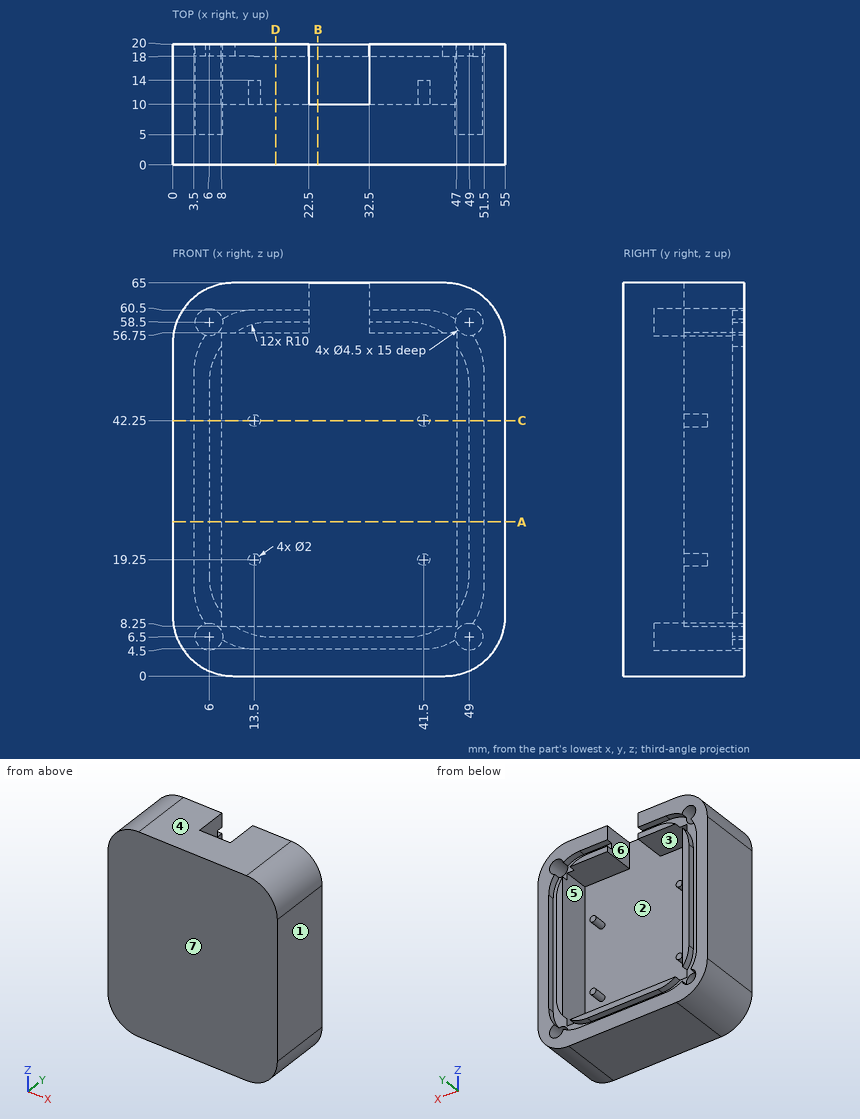
Here's the drawing with two shaded views (mm, measured from the low corner). I have some questions. A direction names the side the tool comes from. Round coordinates to 2 decimals unless told otherwise and drop trailing zeros. Write each loop counter-clockwise with the first axis right and the second up, starting at its lowest first coordinate (ties: lowest second). Pieces come first, ordered by that corner, then holes. Notation, with made-up numbers: M 82.25,41.5 L 93.25,41.5 A28 cw 93.25,78.5 Z; hole C 62.5,-34 d5. An arc over 180 degrees is marked long. Write each question's results on one line, items separated by ' | '. Start each with the question number.
1. On a 3-axis mill with a long thin cutter (end or side, diameter ignored), from which of +Z, -Z, +X, -X, +Y, -Y can I reach the whole of each face in a straight line? I mean the marked faces 5, 6 and 7. Say none if no direction works.
2. Imagine slicing it at A-A on z = 25.5. List the corners of the cut face in (x, y) for me, and give its area (3 significant figures).
3. I need wall thicknesses on L1, parallel to X at y = 14.75, z = 6.5; L2, parallel to Z at x = 49, y = 8.5; L3, parallel to X at y = 19, z = 50. Which ranges of each line are inside material? Lowest first, please. Write a range as from..to.
4. I'm going to push flat-ended pins straight in: pin 1 Ø2 at (x, z) = (6, 5.5) entering from +Y; pin 2 Ø0.6 at (x, z) = (41.5, 19) entering from +Y; pin 3 Ø3.5 at (x, z) = (48, 57.5) entering from +Y. Where does each tip first touch, or does it pass through?
5. Thinking about a two-plate mould opening in Z: for the marked faces 1, 2, 3 and 4, which applies, +Z half, -Z half, draft (parallel to the pull), parting line (faces both ways), or undercut?
6. Imagine slicing it at D-D on x = 17. List the corners of the cut face in (y, z) for me, and give its area (3 significant figures).
7. Imagine slicing it at B-B on x = 24. List the corners of the cut face in (y, z) for me, and give its area (4 significant figures).
8. Imagine slicing it at C-C on z = 42.25. List the corners of the cut face in (x, y) for me, and give its area (3 significant figures).
Result sheet:
1) face 5: +Y | face 6: +Z, +Y | face 7: +Z, -Z, +X, -X, -Y
2) outline: M 0,0 L 55,0 L 55,20 L 51.5,20 L 51.5,18 L 49,18 L 49,20 L 47,20 L 47,10 L 8,10 L 8,20 L 6,20 L 6,18 L 3.5,18 L 3.5,20 L 0,20 Z | area: 700 mm^2
3) L1: x = 0.63..3.75, 8.25..46.75, 51.25..54.37 | L2: z = 0.83..4.25, 8.75..56.25, 60.75..64.17 | L3: x = 0..3.5, 6.11..8, 47..48.89, 51.5..55
4) pin 1: stops at y = 5 | pin 2: stops at y = 14 | pin 3: stops at y = 18
5) face 1: draft | face 2: undercut | face 3: undercut | face 4: +Z half
6) outline: M 0,0 L 20,0 L 20,4.5 L 18,4.5 L 18,6.5 L 20,6.5 L 20,8.25 L 10,8.25 L 10,56.75 L 20,56.75 L 20,58.5 L 18,58.5 L 18,60.5 L 20,60.5 L 20,65 L 0,65 Z | area: 807 mm^2
7) outline: M 0,0 L 20,0 L 20,4.5 L 18,4.5 L 18,6.5 L 20,6.5 L 20,8.25 L 10,8.25 L 10,65 L 0,65 Z | area: 728.5 mm^2
8) outline: M 0,0 L 55,0 L 55,20 L 51.5,20 L 51.5,18 L 49,18 L 49,20 L 47,20 L 47,10 L 42.5,10 L 42.5,14 L 40.5,14 L 40.5,10 L 14.5,10 L 14.5,14 L 12.5,14 L 12.5,10 L 8,10 L 8,20 L 6,20 L 6,18 L 3.5,18 L 3.5,20 L 0,20 Z | area: 716 mm^2
